Geometry: final body of the model. Coordinates: model frame, mm. Coordinates: 2 decimals unless noted, no trailing zeros. Write each loop counter-clockwise with the first axis right and the second up, starting at its lowest first coordinate (ties: lowest second). Pieces come first, ordered by that corner, then holes. Notation, with made-up numbers: (-32, 24.25) - (11, 24.25) arc R27 cw to (11, 51.25) - close; hole circle Ø10 at (-25.75, -22.5). An arc over 180 degrees is marked (long way). Put each result on its own line as item: value.
```python
from build123d import *

# Parameters (mm, degrees)
F0_R     = 7.5
F1_DEPTH = 10


with BuildPart() as f1:
    # F0 (on Right) → F1 (new body)
    with BuildSketch(Plane.YZ):
        Polygon((-21, 0), (73, 0), (101.284271, 28.284271), (135.091675, 37.342938), (149.844361, 92.40071), (78.830278, 133.40071), (19.908802, 117.612748), (-31.709993, 65.993953), (-49.882578, 27.022718), align=None)
        with Locations((0, 44)):
            Circle(F0_R, mode=Mode.SUBTRACT)
        with Locations((27, 44)):
            Circle(F0_R, mode=Mode.SUBTRACT)
        with Locations((54, 44)):
            Circle(F0_R, mode=Mode.SUBTRACT)
        with Locations((108, 44)):
            Circle(F0_R, mode=Mode.SUBTRACT)
        with Locations((0, 74)):
            Circle(F0_R, mode=Mode.SUBTRACT)
        with Locations((27, 74)):
            Circle(F0_R, mode=Mode.SUBTRACT)
        with Locations((54, 74)):
            Circle(F0_R, mode=Mode.SUBTRACT)
        with Locations((81, 74)):
            Circle(F0_R, mode=Mode.SUBTRACT)
        with Locations((108, 74)):
            Circle(F0_R, mode=Mode.SUBTRACT)
        with Locations((54, 104)):
            Circle(F0_R, mode=Mode.SUBTRACT)
        with Locations((81, 104)):
            Circle(F0_R, mode=Mode.SUBTRACT)
        with Locations((108, 104)):
            Circle(F0_R, mode=Mode.SUBTRACT)
    extrude(amount=F1_DEPTH)


solid = f1.part
```
1. Pin query (flat end, axial travel): pin 1 Ø6 at (y, z) = (10, 84) entering from -X; pin 2 Ø1 at (x, y) = (4, 80.5) entering from +Z; pin 3 Ø1 at (x, y) = (6, 57) entering from +Z; pin 4 Ø2 at (x, y) = (8.5, 42.5) entering from +Z. Return the tip coordinate at first contact, or that it passes through.
Answer below:
pin 1: stops at x = 0
pin 2: stops at z = 132.73
pin 3: stops at z = 127.69
pin 4: stops at z = 123.93
2. Section query C-C (z = 44). Return loops of the section in (x, y), then the cut area to 3 significant figures.
Answer below:
outline: (0, -41.97) - (10, -41.97) - (10, -7.5) - (0, -7.5) - close; (0, 7.5) - (10, 7.5) - (10, 19.5) - (0, 19.5) - close; (0, 34.5) - (10, 34.5) - (10, 46.5) - (0, 46.5) - close; (0, 61.5) - (10, 61.5) - (10, 100.5) - (0, 100.5) - close; (0, 115.5) - (10, 115.5) - (10, 136.88) - (0, 136.88) - close
area: 1,190 mm²
3. Mould query, pull axis Y, two halves, no side actions, for faces 1 (the flat face through (4.93, -5.539, 92.165)), 2 (the flat face through (4.93, 117.95, 32.75)), 3 (the flat face through (10, 49, 68)), 4 (the cylindrical face through (4.93, 52.37, 96.68)). Classes: +Y half, -Y half, draft (parallel to the pull), parting line (faces both ways), or undercut.
Answer below:
face 1: -Y half
face 2: +Y half
face 3: draft
face 4: undercut
4. Section query A-A (x = 3.75). Count the separate pieces of the cut face and the enclosed holes in it, then the cut area to 3 significant figures.
Answer below:
separate pieces: 1
enclosed holes: 12
area: 16,000 mm²
5. Section query D-D (y = 0). Return loops of the section in (x, z).
Answer below:
outline: (0, 0) - (10, 0) - (10, 36.5) - (0, 36.5) - close; (0, 51.5) - (10, 51.5) - (10, 66.5) - (0, 66.5) - close; (0, 81.5) - (10, 81.5) - (10, 97.7) - (0, 97.7) - close
6. Section query B-B (y = 55). Return loops of the section in (x, z).
Answer below:
outline: (0, 0) - (10, 0) - (10, 36.57) - (0, 36.57) - close; (0, 51.43) - (10, 51.43) - (10, 66.57) - (0, 66.57) - close; (0, 81.43) - (10, 81.43) - (10, 96.57) - (0, 96.57) - close; (0, 111.43) - (10, 111.43) - (10, 127.02) - (0, 127.02) - close
7. Ray query, probe 1 along Z at (x, y) = (6.25, 27); probe 2 along Z at (x, y) = (8, 0); probe 3 along Z at (x, y) = (0.75, 57). Return the intervals inside material, ascending. Write a range as from..to.
Answer below:
probe 1: z = 0..36.5, 51.5..66.5, 81.5..119.51
probe 2: z = 0..36.5, 51.5..66.5, 81.5..97.7
probe 3: z = 0..37.13, 50.87..67.13, 80.87..97.13, 110.87..127.55
